Source: CAD feature listing. Evaluate the final solid. Frame: model axes, mm. A direction names the side the tool comes from. Round coordinates to 2 decimals unless told otherwise and drop trailing zeros. Write each loop counter-clockwise with the first axis right and the second up, starting at its lowest first coordinate (ties: lowest second). Pieces come first, ordered by that corner, then holes. Notation, with made-up numbers: M -8.5,71 L 26.5,71 A25 cw 26.5,90 Z; hole C -11,54.25 d11. An arc over 180 degrees is marked long. Answer in a Markdown table with one row per item.
from build123d import *

# Parameters (mm, degrees)
BOSS_EXTRUDE1_DEPTH = 10
BOSS_EXTRUDE2_START = 10
BOSS_EXTRUDE2_DEPTH = 86
BOSS_EXTRUDE3_DEPTH = 7


with BuildPart() as part:
    # Sketch1 → Boss-Extrude1 (new body)
    # profile 1 of 2: a face of its own
    with BuildSketch(Plane.XY):
        Polygon((42, -8.35431943), (42, 8.35431943), (35.605880731, 23.791088889), (23.791088889, 35.605880731), (8.35431943, 42), (-8.35431943, 42), (-23.791088889, 35.605880731), (-35.605880731, 23.791088889), (-42, 8.35431943), (-42, -8.35431943), (-35.605880731, -23.791088889), (-23.791088889, -35.605880731), (-8.35431943, -42), (8.35431943, -42), (23.791088889, -35.605880731), (35.605880731, -23.791088889), align=None)
        Polygon((27.128290081, 18.126543915), (18.126543915, 27.128290081), (6.365195756, 32), (-6.365195756, 32), (-18.126543915, 27.128290081), (-27.128290081, 18.126543915), (-32, 6.365195756), (-32, -6.365195756), (-27.128290081, -18.126543915), (-18.126543915, -27.128290081), (-6.365195756, -32), (6.365195756, -32), (18.126543915, -27.128290081), (27.128290081, -18.126543915), (32, -6.365195756), (32, 6.365195756), align=None, mode=Mode.SUBTRACT)
    # profile 2 of 2: a face of its own
    with BuildSketch(Plane.XY):
        Polygon((32, 6.365195756), (27.128290081, 18.126543915), (18.126543915, 27.128290081), (6.365195756, 32), (-6.365195756, 32), (-18.126543915, 27.128290081), (-27.128290081, 18.126543915), (-32, 6.365195756), (-32, -6.365195756), (-27.128290081, -18.126543915), (-18.126543915, -27.128290081), (-6.365195756, -32), (6.365195756, -32), (18.126543915, -27.128290081), (27.128290081, -18.126543915), (32, -6.365195756), align=None)
    extrude(amount=BOSS_EXTRUDE1_DEPTH)

    # Sketch1<5> → Boss-Extrude2 (add)
    with BuildSketch(Plane.XY.offset(BOSS_EXTRUDE2_START)):
        Polygon((42, -8.35431943), (42, 8.35431943), (35.605880731, 23.791088889), (23.791088889, 35.605880731), (8.35431943, 42), (-8.35431943, 42), (-23.791088889, 35.605880731), (-35.605880731, 23.791088889), (-42, 8.35431943), (-42, -8.35431943), (-35.605880731, -23.791088889), (-23.791088889, -35.605880731), (-8.35431943, -42), (8.35431943, -42), (23.791088889, -35.605880731), (35.605880731, -23.791088889), align=None)
        Polygon((27.128290081, 18.126543915), (18.126543915, 27.128290081), (6.365195756, 32), (-6.365195756, 32), (-18.126543915, 27.128290081), (-27.128290081, 18.126543915), (-32, 6.365195756), (-32, -6.365195756), (-27.128290081, -18.126543915), (-18.126543915, -27.128290081), (-6.365195756, -32), (6.365195756, -32), (18.126543915, -27.128290081), (27.128290081, -18.126543915), (32, -6.365195756), (32, 6.365195756), align=None, mode=Mode.SUBTRACT)
    extrude(amount=BOSS_EXTRUDE2_DEPTH)

    # Sketch3 → Boss-Extrude3 (add, symmetric)
    with BuildSketch(Plane(origin=(0, 0, 0), x_dir=(0, 0, -1), z_dir=(1, 0, 0))):
        Polygon((-86, 42), (-86, 67), (-31, 67), (-20, 42), (-26.555120136, 42), (-34.915120136, 61), (-80, 61), (-80, 42), align=None)
    extrude(amount=BOSS_EXTRUDE3_DEPTH, both=True)


solid = part.part
Q1. Section B-B (z = 46). State how many separate pieces and enclosed holes the cut face has, and give its area (3 significant figures).
Solutions:
| item | result |
|---|---|
| separate pieces | 2 |
| enclosed holes | 1 |
| area | 2,440 mm2 |
Q2. Pull-direction query (Y, two-part tool) for faces 1 (the flat face through (12.33, 29.53, 52.4)), 2 (the flat face through (0, 32, 52)), 3 (the flat face through (-29.781, -29.616, 47.328)), 4 (the flat face through (7, 63, 53)); classes: pulls with the +Y half, pulls with the -Y half, needs draft (parallel to the pull), parting line crosses it, or undercut.
Solutions:
| item | result |
|---|---|
| face 1 | undercut |
| face 2 | undercut |
| face 3 | pulls with the -Y half |
| face 4 | needs draft |
Q3. Section C-C (y = 1). Return loops of the section in (x, z).
Solutions:
| item | result |
|---|---|
| outline | M -42,0 L 42,0 L 42,96 L 32,96 L 32,10 L -32,10 L -32,96 L -42,96 Z |
Q4. Material intervals for probe 1 along Z at (x, y) = (8, -4); probe 2 along X at (y, z) = (48.5, 24); probe 3 along X at (y, z) = (-21, 92.5), sorted ascending.
Solutions:
| item | result |
|---|---|
| probe 1 | z = 0 to 10 |
| probe 2 | x = -7 to 7 |
| probe 3 | x = -36.76 to -24.25, 24.25 to 36.76 |
Q5. Access query for faces 5 (the flat face through (-7, 63, 53)), 6 (the flat face through (38.76, -16.18, 47.33)), 7 (the flat face through (-32, 0, 52)), 8 (the flat face through (16.18, 38.76, 47.33)), 9 (the flat face through (0, 54, 86)). Directions: +Z, -Z, +X, -X, +Y, -Y. A direction counts if a zero-diameter tool reaches every point of the face in a straight line with its end or side. Return the directions, or none.
Solutions:
| item | result |
|---|---|
| face 5 | +Z, -Z, -X, +Y |
| face 6 | +Z, -Z, +X, -Y |
| face 7 | +Z |
| face 8 | +Z, -Z, +X, +Y |
| face 9 | +Z, +X, -X, +Y |
Q6. Section A-A (x = 0.5). Return loops of the section in (y, z), and give its area (3 significant figures).
Solutions:
| item | result |
|---|---|
| outline | M -42,0 L 42,0 L 42,20 L 67,31 L 67,86 L 42,86 L 42,96 L 32,96 L 32,10 L -32,10 L -32,96 L -42,96 Z; hole M 42,26.56 L 61,34.92 L 61,80 L 42,80 Z |
| area | 3,140 mm2 |
Q7. Contact query for flat-ended pins moving along their axis: pin 1 Ø4 at (x, y) = (6, -4) entering from +Z; pin 2 Ø1 at (y, z) = (20.5, 78.5) entering from +X; pin 3 Ø5 at (x, z) = (-15, 39.5) entering from +Y; pin 4 Ø12 at (x, y) = (-17.5, 55) entering from -Z. Output: stop coordinate, or through.
Solutions:
| item | result |
|---|---|
| pin 1 | stops at z = 10 |
| pin 2 | stops at x = 37.18 |
| pin 3 | stops at y = 40.28 |
| pin 4 | passes through |
